Check sheet for the modelled part. Datum: model origin and axes. Units: mm. Round coordinates to 2 decimals unless told otherwise and drop trailing zeros. Order: outer loops, then holes, each group sorted by start corner. A loop starts at its lowest first (then second) coordinate and runs counter-clockwise, first axis right, second up. Notation, with made-up numbers: (43, 51) -> (61, 51) arc R27 ccw to (61, 90) -> close; hole circle Ø6 at (62.25, -21.75). An arc over 180 degrees is marked (long way). Use CSV: the item, a comma, the result in double quotes.
Autodesk Inventor part; units mm, degrees
ref_plane "YZ Plane" through (0, 0, 0) normal (1, 0, 0) x (0, 1, 0)
ref_plane "XZ Plane" through (0, 0, 0) normal (0, 1, 0) x (-1, 0, 0)
ref_plane "XY Plane" through (0, 0, 0) normal (0, 0, 1) x (1, 0, 0)
sketch "Sketch1" plane through (0, 0, 0) normal (0, 1, 0) x (-1, 0, 0)
  line L0 (127, 143.8324) -> (0, 143.8324)
  line L1 (0, 143.8324) -> (0, -160.9676)
  line L2 (0, -160.9676) -> (127, -160.9676)
  line L3 (127, -160.9676) -> (127, 143.8324)
  line L4 (0, -160.9676) -> (12.7, -160.9676)
  line L5 (12.7, -160.9676) -> (12.7, -8.5676)
  line L6 (12.7, -8.5676) -> (0, -8.5676)
  line L7 (0, -8.5676) -> (0, -160.9676)
  line L8 (12.7, -8.5676) -> (88.9, 93.0324)
  line L9 (0, -8.5676) -> (76.2, 93.0324)
  line L10 (127, 143.8324) -> (76.2, 143.8324)
  line L11 (76.2, 143.8324) -> (76.2, 93.0324)
  line L12 (88.9, 93.0324) -> (127, 93.0324)
  line L13 (127, 93.0324) -> (127, 143.8324)
  line L14 (88.9, 93.0324) -> (88.9, 143.8324)
  point P0 (0, 0)
  point P1 (114.3, 143.8324)
  dimension "d0" = 304.8
  dimension "d1" = 127
  dimension "d2" = 12.7
  dimension "d3" = 152.4
  dimension "d16" = 50.8
  dimension "d17" = 0
  dimension "d18" = 12.7
extrude "Extrusion1" add sketch "Sketch1" along normal blind 25.4 contours L14 L8 L6 L9 L11 L0 | L5 L2 L1 L6
sketch "Sketch2" plane through (0, 0, -8.5676) normal (1, 0, 0) x (0, 0, -1)
  circle A0 centre (127, 12.7) radius 3.175
  line L0 (0, 0) -> (152.4, 0)
  line L1 (152.4, 0) -> (152.4, 25.4)
  point P0 (-8.5676, 0)
  dimension "d6" = 6.35
  dimension "d7" = 12.7
  dimension "d8" = 25.4
extrude "Extrusion2" cut sketch "Sketch2" against normal through all
sketch "Sketch4" plane through (-76.2, 0, 143.8324) normal (1, 0, 0) x (0, 0, -1)
  circle A0 centre (25.4, 12.7) radius 3.175
  line L0 (0, 0) -> (50.8, 0)
  line L1 (0, 0) -> (0, 25.4)
  point P0 (143.8324, 0)
  dimension "d19" = 6.35
  dimension "d20" = 12.7
  dimension "d21" = 25.4
extrude "Extrusion4" cut sketch "Sketch4" against normal through all
properties part number "arm2"
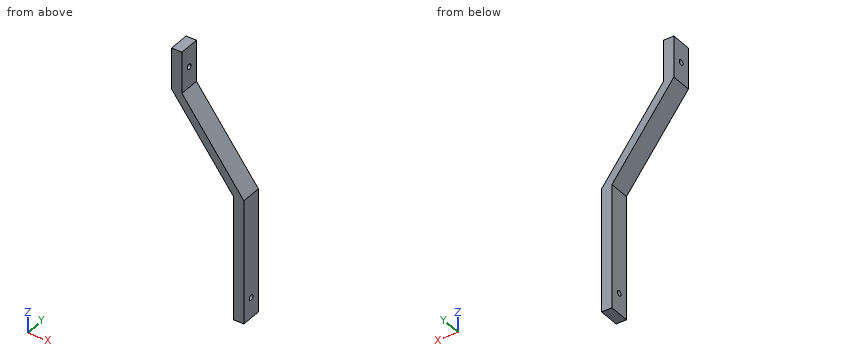
Q1. Go/stop test with flat-tipped pins: pin 1 (2 mm diameter, centred on y = 4, z = 26.5, fed in from +X); pin 2 (1.5 mm diameter, centred on x = -38, y = 15, fed in from -Z); pin 3 (2 mm diameter, centred on y = 10, z = 91, fed in from +X); pin 4 (1 mm diameter, centred on y = 12.5, z = -30.5, fed in from +X). Record where each tip stops, or that it passes through.
Result sheet:
pin 1,"stops at x = -25.55"
pin 2,"stops at z = 24.17"
pin 3,"stops at x = -73.93"
pin 4,"stops at x = 0"
Q2. Sectioned sample at B-B, the plane x = -10. Enter the section's corners in (y, z) (3 decimals), then the cut area to 3 significant figures.
Result sheet:
outline,"(0, -160.968) -> (25.4, -160.968) -> (25.4, 4.766) -> (0, 4.766) -> close; hole circle Ø6.35 at (12.7, -135.568)"
area,"4,180 mm^2"
Q3. Sectioned sample at C-C, the plane z = -55. Enter the section's corners in (x, y), then the cut area to 3 significant figures.
Result sheet:
outline,"(-12.7, 0) -> (0, 0) -> (0, 25.4) -> (-12.7, 25.4) -> close"
area,"323 mm^2"
Q4. Sectioned sample at A-A, the plane y = 12.7. Enter the section's corners in (x, z).
Result sheet:
outline,"(-88.9, 93.03) -> (-12.7, -8.57) -> (-12.7, -132.39) -> (0, -132.39) -> (0, -8.57) -> (-76.2, 93.03) -> (-76.2, 115.26) -> (-88.9, 115.26) -> close; (-88.9, 121.61) -> (-76.2, 121.61) -> (-76.2, 143.83) -> (-88.9, 143.83) -> close; (-12.7, -160.97) -> (0, -160.97) -> (0, -138.74) -> (-12.7, -138.74) -> close"
Q5. Scan lines: L1, parallel to X at y = 21, z = -14; L2, parallel to X at y = 7.75, z = -1; L3, parallel to Z at x = -10, y = 24. Record each from-to range of solid material in increasing order.
Result sheet:
L1,"x = -12.7 to 0"
L2,"x = -18.38 to -5.68"
L3,"z = -160.97 to 4.77"
Q6. Sectioned sample at D-D, the plane x = -30. Enter the section's corners in (y, z).
Result sheet:
outline,"(0, 14.5) -> (25.4, 14.5) -> (25.4, 31.43) -> (0, 31.43) -> close"
